Study the drawing (mm; zero at the part's minimum x, y, z) and answer. A direction names the side the tool comes from. Round coordinates to 2 decimals unless told otherwise and drop trailing zeros. Write each loop counter-clockwise with the first axis right and the second up, starting at its lowest first coordinate (ties: lowest second). Pieces come first, ordered by that corner, then holes. Notation, with made-up numbers: M 62,22 L 91,22 A7 ccw 91,30 Z; hole C -10.5,-36.75 d4. An arc over 180 degrees is marked long. Put each result on its own line as item: value. Start each with the question number.
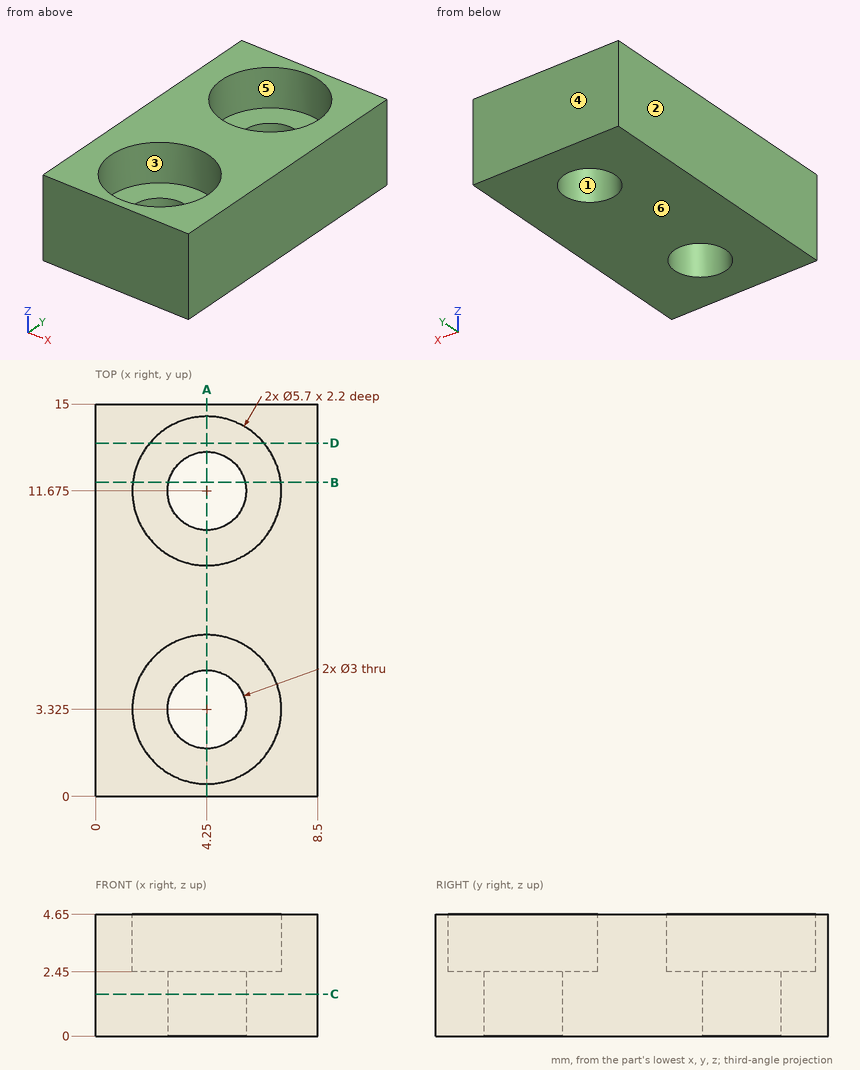
Item 1: Determine the mould class of the marked faces 1, 2, 3 and 4 for opening direction X: released by +X, released by -X, zero draft, split by the parting line, or undercut.
Item 2: Section C-C (z = 1.6) is taken. Give the vertices of the cut face in (x, y) (3 decimals), and give its area (3 significant figures).
Item 3: Section B-B (y = 12) is taken. Give the vertices of the cut face in (x, z).
Item 4: Which of the six approach directions +Z, -Z, +X, -X, +Y, -Y give full straight-line access (tool end or side, diameter ignored) to the marked faces 5 and 6?
Item 5: Flat-ended cylindrical pins translate along their axes: pin 1 (2.5 mm diameter, centred on x = 4.25, y = 11.675, fed in from -Z); pin 2 (5 mm diameter, centred on x = 4.25, y = 3.325, fed in from +Z). Find the tip coordinate at first contact, or state that the pin passes through.
Item 6: Section A-A (x = 4.25) is taken. Give the vertices of the cut face in (y, z) (3 decimals).
Item 7: Section D-D (y = 13.5) is taken. Give the vertices of the cut face in (x, z).
Item 8: Consider line 1 along Y through (x, z) = (4.25, 3.9) (3 decimals); line 2 along Y through (x, z) = (4.25, 1.3) (3 decimals); line 3 along X through (y, z) = (5.75, 3.3). Determine where each line is inside the solid, lowest interval first. Write a range as [from, to].
Output values:
1. face 1: undercut
1. face 2: released by -X
1. face 3: undercut
1. face 4: zero draft
2. outline: M 0,0 L 8.5,0 L 8.5,15 L 0,15 Z; hole C 4.25,3.325 d3; hole C 4.25,11.675 d3
2. area: 113 mm^2
3. outline: M 0,0 L 2.79,0 L 2.79,2.45 L 1.42,2.45 L 1.42,4.65 L 0,4.65 Z; M 5.71,0 L 8.5,0 L 8.5,4.65 L 7.08,4.65 L 7.08,2.45 L 5.71,2.45 Z
4. face 5: +Z
4. face 6: -Z, +X, -X, +Y, -Y
5. pin 1: passes through
5. pin 2: stops at z = 2.45
6. outline: M 0,0 L 1.825,0 L 1.825,2.45 L 0.475,2.45 L 0.475,4.65 L 0,4.65 Z; M 4.825,0 L 10.175,0 L 10.175,2.45 L 8.825,2.45 L 8.825,4.65 L 6.175,4.65 L 6.175,2.45 L 4.825,2.45 Z; M 13.175,0 L 15,0 L 15,4.65 L 14.525,4.65 L 14.525,2.45 L 13.175,2.45 Z
7. outline: M 0,0 L 8.5,0 L 8.5,4.65 L 6.44,4.65 L 6.44,2.45 L 2.06,2.45 L 2.06,4.65 L 0,4.65 Z
8. line 1: y = [0, 0.475], [6.175, 8.825], [14.525, 15]
8. line 2: y = [0, 1.825], [4.825, 10.175], [13.175, 15]
8. line 3: x = [0, 2.75], [5.75, 8.5]
